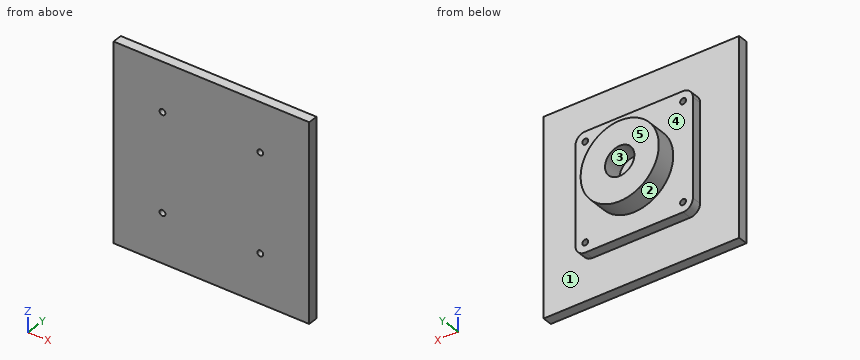
Autodesk Inventor part; units mm, degrees
ref_plane "YZ Plane" through (0, 0, 0) normal (1, 0, 0) x (0, 1, 0)
ref_plane "XZ Plane" through (0, 0, 0) normal (0, 1, 0) x (-1, 0, 0)
ref_plane "XY Plane" through (0, 0, 0) normal (0, 0, 1) x (1, 0, 0)
sketch "Sketch1" plane through (0, 0, 0) normal (0, 1, 0) x (-1, 0, 0)
  line L0 (-100, 100) -> (100, 100)
  line L1 (100, 100) -> (100, -100)
  line L2 (100, -100) -> (-100, -100)
  line L3 (-100, -100) -> (-100, 100)
  line L4 (-100, 100) -> (100, -100) construction
  line L5 (100, 100) -> (-100, -100) construction
  point P0 (0, 0)
  dimension "d0" = 200
  dimension "d1" = 200
extrude "Extrusion1" add sketch "Sketch1" along normal blind 10
sketch "Sketch2" plane through (0, 10, 0) normal (0, 1, 0) x (1, 0, 0)
  line L0 (60, -60) -> (-60, -60)
  line L1 (-60, -60) -> (-60, 60)
  line L2 (-60, 60) -> (60, 60)
  line L3 (60, 60) -> (60, -60)
  line L4 (60, -60) -> (-60, 60) construction
  line L5 (-60, -60) -> (60, 60) construction
  point P0 (0, 0)
  dimension "d4" = 120
  dimension "d5" = 120
extrude "Extrusion2" add sketch "Sketch2" along normal blind 10
fillet "Fillet1" radius 10 4 edges at (60, 15, 60) (60, 15, -60) (-60, 15, 60) (-60, 15, -60)
sketch "Sketch3" plane through (0, 20, 0) normal (0, 1, 0) x (1, 0, 0)
  circle A0 centre (0, 0) radius 15
  circle A1 centre (0, 0) radius 40
  dimension "d9" = 30
  dimension "d19" = 80
extrude "Extrusion3" add sketch "Sketch3" along normal blind 20
sketch "Sketch4" plane through (0, 20, 0) normal (0, 1, 0) x (1, 0, 0)
  arc A0 (60, 50) -> (50, 60) centre (50, 50) ccw
  arc A1 (50, -60) -> (60, -50) centre (50, -50) ccw
  arc A2 (-60, -50) -> (-50, -60) centre (-50, -50) ccw
  arc A3 (-50, 60) -> (-60, 50) centre (-50, 50) ccw
  point P0 (0, 0)
hole "Hole1" at (50, 20, 50) at (-50, 20, 50) at (50, 20, -50) at (-50, 20, -50) direction (0, -1, 0) diameter 6 end through all
properties part number "Base Plate 2"
For this review, take the finished solid that the model builds, in its own axes (mm). Face numbers are marked on the shaded views. A direction names the side the tool comes from. Give positions to 0.01 mm unless a question says otherwise; leave off trailing zeros. Order: outer loops, then holes, each group sorted by start corner. A loop starts at its lowest first (then second) coordinate and runs counter-clockwise, first axis right, second up. Notation, with made-up numbers: (61.5, -1.75) -> (116.5, -1.75) arc R18 ccw to (116.5, 26.25) -> close; hole circle Ø7 at (10, 75). An arc over 180 degrees is marked (long way). Write item = value, one per line.
1) To check wall thickness, follow L1, parallel to Z at x = -50, y = 11; L2, parallel to X at y = 6.5, z = -50. State the ranges of each line that lie inside material, in increasing order. Write a range as from..to.
Findings:
L1 = -60..-53, -47..47, 53..60
L2 = -100..-53, -47..47, 53..100
2) For the marked faces 4 and 5, list the 3-axis set-ups (+Z, -Z, +X, -X, +Y, -Y) from which the entire face can be reached by the end or side of a thin tool; tool diameter is ignored.
Findings:
face_4 = +Y
face_5 = +Z, -Z, +X, -X, +Y
3) We need section B-B, the plane z = 0. Give the boundary of the cut face in (x, y).
Findings:
outline = (-100, 0) -> (100, 0) -> (100, 10) -> (60, 10) -> (60, 20) -> (40, 20) -> (40, 40) -> (15, 40) -> (15, 20) -> (-15, 20) -> (-15, 40) -> (-40, 40) -> (-40, 20) -> (-60, 20) -> (-60, 10) -> (-100, 10) -> close
4) Draft analysis for pull direction Z (two halves, no side actions). For the marked faces 1, 2 and 3, state which applies: pulls with the +Z half, pulls with the -Z half, needs draft (parallel to the pull), parting line crosses it, or undercut.
Findings:
face_1 = needs draft
face_2 = parting line crosses it
face_3 = undercut
5) We need section D-D, the plane y = 36.5. Give the boundary of the cut face in (x, z), and give its area (3 significant figures).
Findings:
outline = circle Ø80 at (0, 0); hole circle Ø30 at (0, 0)
area = 4,320 mm^2
6) We need section C-C, the plane x = 30. Give the boundary of the cut face in (y, z), and give its area (3 significant figures).
Findings:
outline = (0, -100) -> (10, -100) -> (10, -60) -> (20, -60) -> (20, -26.46) -> (40, -26.46) -> (40, 26.46) -> (20, 26.46) -> (20, 60) -> (10, 60) -> (10, 100) -> (0, 100) -> close
area = 4,260 mm^2
7) Insertion check: pin 1 (6 mm diameter, centred on x = 53, z = -8.5, fed in from +Y); pin 2 (4 mm diameter, centred on y = 13.5, z = 50, fed in from -X); pin 3 (1.5 mm diameter, centred on x = 48.5, y = 19.5, fed in from +Z). Each pin has a flat end and moves straight along its axis. Give the tip position at first contact, or say it passes through.
Findings:
pin_1 = 20
pin_2 = -60
pin_3 = 60
8) We need section A-A, the plane y = 14.5. Give the boundary of the cut face in (x, z), and give its area (3 significant figures).
Findings:
outline = (-60, -50) arc R10 ccw to (-50, -60) -> (50, -60) arc R10 ccw to (60, -50) -> (60, 50) arc R10 ccw to (50, 60) -> (-50, 60) arc R10 ccw to (-60, 50) -> close; hole circle Ø6 at (-50, -50); hole circle Ø6 at (-50, 50); hole circle Ø6 at (50, -50); hole circle Ø6 at (50, 50)
area = 14,200 mm^2
